from build123d import *

# Parameters (mm, degrees)
RESSALTO_EXTRUS_O1_DEPTH = 3
ESBO_O2_R                = 4
CORTE_EXTRUS_O1_DEPTH    = 219.690902409


with BuildPart() as part:
    # Esboço1 → Ressalto-extrusão1 (new body)
    with BuildSketch(Plane(origin=(0, 0, 0), x_dir=(1, 0, 0), z_dir=(0, 1, 0))):
        Polygon((97.255710926, -182.75), (120.079758063, -92.387934551), (120.079758063, 97.512065449), (35.4, 180.55), (-35.4, 180.55), (-119.989494029, 104.35), (-119.989494029, -104.35), (-98.094289074, -182.75), align=None)
    extrude(amount=RESSALTO_EXTRUS_O1_DEPTH)

    # Esboço2 → Corte-extrusão1 (cut, through all)
    with BuildSketch(Plane(origin=(0, 3, 0), x_dir=(1, 0, 0), z_dir=(0, 1, 0))):
        with Locations(Location((24.579758063, -165.65, 0), (0, 0, 270))):
            Circle(ESBO_O2_R)
        with Locations(Location((-20.420241937, -165.65, 0), (0, 0, 270))):
            Circle(ESBO_O2_R)
    extrude(amount=-CORTE_EXTRUS_O1_DEPTH, mode=Mode.SUBTRACT)


solid = part.part
For this review, take the finished solid that the model builds, in its own axes (mm). Coordinates: 2 decimals unless noted, no trailing zeros. Loops run counter-clockwise (first coordinate to the right, second up) from the corner with the lowest first, then second, coordinate; pieces in that order, holes last. Notation, with made-up numbers: (41, 60.25) - (72, 60.25) arc R26 ccw to (72, 94.25) - close; hole circle Ø11 at (52.5, 67). An arc over 180 degrees is marked (long way). Use a Markdown table: item, result. Add a question column.
Item 1: For line 1 (X direction, y = 1.55, z = 165.65); line 2 (Z direction, x = -23, y = 0.45); line 3 (Z direction, x = -38.5, y = 0.9), list the stretches that pass through material, from the lowest coordinate up.
Item 2: Mouldability with a two-part tool opening along X and no side actions: class faces 1 (the face through (108.51, 1.48, 138.2)), 2 (the face through (-77.103, 1.479, -142.983)), 3 (the face through (-17.72, 1.52, 162.7)) as pulls with the +X half, pulls with the -X half, needs draft (parallel to the pull), parting line crosses it, or undercut.
Item 3: Insertion check: pin 1 Ø7 at (x, z) = (-20.42, 165.65) entering from -Y. The pin has a flat end and moves straight along its axis. Give the tip position at first contact, or say it passes through.
Item 4: We need section C-C (x = -74). Give the boundary of the cut face in (y, z).
Item 5: We need section A-A (z = 165.65). Give the boundary of the cut face in (x, y).
Item 6: We need section D-D (x = 41). Give the boundary of the cut face in (y, z).
Item 7: We need section B-B (y = 1.15). Give the boundary of the cut face in (x, z), and give its area (3 significant figures).
Results list:
| question | item | result |
|---|---|---|
| 1 | line 1 | x = -102.87 to -24.42, -16.42 to 20.58, 28.58 to 101.57 |
| 1 | line 2 | z = -180.55 to 162.59, 168.71 to 182.75 |
| 1 | line 3 | z = -177.76 to 182.75 |
| 2 | face 1 | pulls with the +X half |
| 2 | face 2 | pulls with the -X half |
| 2 | face 3 | undercut |
| 3 | pin 1 | passes through |
| 4 | outline | (0, -145.78) - (3, -145.78) - (3, 182.75) - (0, 182.75) - close |
| 5 | outline | (-102.87, 0) - (-24.42, 0) - (-24.42, 3) - (-102.87, 3) - close; (-16.42, 0) - (20.58, 0) - (20.58, 3) - (-16.42, 3) - close; (28.58, 0) - (101.57, 0) - (101.57, 3) - (28.58, 3) - close |
| 6 | outline | (0, -175.06) - (3, -175.06) - (3, 182.75) - (0, 182.75) - close |
| 7 | outline | (-119.99, -104.35) - (-35.4, -180.55) - (35.4, -180.55) - (120.08, -97.51) - (120.08, 92.39) - (97.26, 182.75) - (-98.09, 182.75) - (-119.99, 104.35) - close; hole circle Ø8 at (-20.42, 165.65); hole circle Ø8 at (24.58, 165.65) |
| 7 | area | 78,500 mm^2 |
